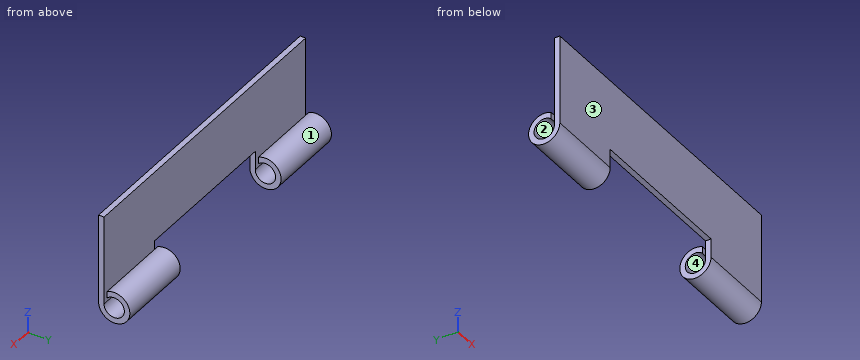
from build123d import *

# Parameters (mm, degrees)
SKETCH1_W           = 50.8
SKETCH1_H           = 15.875
BOSS_EXTRUDE1_DEPTH = 0.889
SKETCH3_W           = 7.62
SKETCH3_H           = 12.7
CUT_EXTRUDE1_DEPTH  = 51.8
BOSS_EXTRUDE6_DEPTH = 12.7
BOSS_EXTRUDE7_START = -25.4
BOSS_EXTRUDE7_DEPTH = 12.7


with BuildPart() as part:
    # Sketch1 → Boss-Extrude1 (new body)
    with BuildSketch(Plane(origin=(0, 0, 0), x_dir=(1, 0, 0), z_dir=(0, 1, 0))):
        with Locations((25.4, 7.9375)):
            Rectangle(SKETCH1_W, SKETCH1_H)
    extrude(amount=BOSS_EXTRUDE1_DEPTH)

    # Sketch3 → Cut-Extrude1 (cut, through all)
    with BuildSketch(Plane(origin=(50.8, 0, 0), x_dir=(0, 0, -1), z_dir=(1, 0, 0))):
        with Locations((0.635, -0.009678267)):
            Rectangle(SKETCH3_W, SKETCH3_H)
    extrude(amount=-CUT_EXTRUDE1_DEPTH, mode=Mode.SUBTRACT)

    # Sketch4 → Boss-Extrude6 (add)
    with BuildSketch(Plane(origin=(38.1, 0, 0), x_dir=(0, 0, -1), z_dir=(1, 0, 0))):
        with BuildLine():
            Line((15.875, 0.889), (18.915054155, 0.889))
            ThreePointArc((18.915054155, 0.889), (19.562629634, 4.058699114), (17.723688552, 1.397))
            Line((17.723688552, 1.397), (16.646761626, 1.397))
            ThreePointArc((16.646761626, 1.397), (20.247041392, 4.702732068), (18.915054155, 0))
            Line((18.915054155, 0), (15.875, 0))
            Line((15.875, 0), (15.875, 0.889))
        make_face()
    extrude(amount=BOSS_EXTRUDE6_DEPTH)

    # Sketch4<4> → Boss-Extrude7 (add)
    with BuildSketch(Plane(origin=(38.1, 0, 0), x_dir=(0, 0, -1), z_dir=(1, 0, 0)).offset(BOSS_EXTRUDE7_START)):
        with BuildLine():
            Line((15.875, 0.889), (18.915054155, 0.889))
            ThreePointArc((18.915054155, 0.889), (19.562629634, 4.058699114), (17.723688552, 1.397))
            Line((17.723688552, 1.397), (16.646761626, 1.397))
            ThreePointArc((16.646761626, 1.397), (20.247041392, 4.702732068), (18.915054155, 0))
            Line((18.915054155, 0), (15.875, 0))
            Line((15.875, 0), (15.875, 0.889))
        make_face()
    extrude(amount=-BOSS_EXTRUDE7_DEPTH)


solid = part.part
Work out the finished part from the listing and answer in its coordinate system (mm). Face numbers are marked on the shaded views. Give positions to 0.01 mm unless a question says otherwise; leave off trailing zeros. Loops run counter-clockwise (first coordinate to the right, second up) from the corner with the lowest first, then second, coordinate; pieces in that order, holes last. Notation, with made-up numbers: M 74.5,-37.5 L 85.5,-37.5 A14 cw 85.5,-16.5 Z; hole C 11.5,25 d1. An arc over 180 degrees is marked long. Use CSV: the item, a comma, the result in double quotes.
1) Consider L1, parallel to Z at x = 7, y = 2.54; L2, parallel to Y at x = 47, z = -14.5; L3, parallel to Y at x = 10.5, z = -19.5. Determine where each line is inside the solid, lowest interval first.
Answer:
L1,"-21.46 to -20.57, -17.26 to -16.38"
L2,"0 to 0.89"
L3,"0.07 to 1, 4.08 to 5.01"
2) Find section A-A on y = 2.54. Write down the section's boundary in (x, z).
Answer:
outline,"M 0,-21.46 L 12.7,-21.46 L 12.7,-20.57 L 0,-20.57 Z; M 0,-17.26 L 12.7,-17.26 L 12.7,-16.38 L 0,-16.38 Z; M 38.1,-21.46 L 50.8,-21.46 L 50.8,-20.57 L 38.1,-20.57 Z; M 38.1,-17.26 L 50.8,-17.26 L 50.8,-16.38 L 38.1,-16.38 Z"
3) Find section B-B on z = -20. Write down the section's boundary in (x, y), plus the area to 3 significant figures.
Answer:
outline,"M 0,0.24 L 12.7,0.24 L 12.7,1.3 L 0,1.3 Z; M 0,3.78 L 12.7,3.78 L 12.7,4.84 L 0,4.84 Z; M 38.1,0.24 L 50.8,0.24 L 50.8,1.3 L 38.1,1.3 Z; M 38.1,3.78 L 50.8,3.78 L 50.8,4.84 L 38.1,4.84 Z"
area,"53.4 mm^2"
4) Find section C-C on x = 4. Write down the section's boundary in (y, z) (3 decimals).
Answer:
outline,"M 0,-18.915 A2.54 ccw long 1.397,-16.647 L 1.397,-17.724 A1.651 cw long 0.889,-18.915 L 0.889,-4.445 L 0,-4.445 Z"
5) Given P1, Ø0.5, axis at x = 5, z = -17, coming from the -Y side; P2, Ø7, axis at x = 31.5, z = -14.5, coming from the +Y side; P3, Ø1.5, axis at x = 27.5, y = 1.5, coming from the -Z side (3 decimals), each flat-ended and moving along its own axis, determine where each tip first touches the part or whether it passes through.
Answer:
P1,"y = 0"
P2,"y = 0.89"
P3,"z = -15.875"
6) Determine the mould class of the marked faces 1, 2, 3 and 4 for opening direction Z: released by +Z, released by -Z, zero draft, split by the parting line, or undercut.
Answer:
face 1,"split by the parting line"
face 2,"undercut"
face 3,"zero draft"
face 4,"undercut"
7) Find section D-D on x = 28. Write down the section's boundary in (y, z) (3 decimals), plus the area to 3 significant figures.
Answer:
outline,"M 0,-15.875 L 0.889,-15.875 L 0.889,-4.445 L 0,-4.445 Z"
area,"10.2 mm^2"
